The model under review builds one solid part; all positions refer to its coordinate system, in mm. A direction names the side the tool comes from. Give positions to 0.01 mm unless a question says otherwise; leave off trailing zeros. Write each loop counter-clockwise with the first axis right and the second up, starting at its lowest first coordinate (ties: lowest second). Pieces come first, ordered by that corner, then holes. Notation, with made-up numbers: (-9, -27) - (10, -27) arc R26 cw to (10, 1) - close; hole circle Ø9 at (-18, -37.75). An arc over 180 degrees is marked (long way). Write item = value, one per line.
```python
from build123d import *

# Parameters (mm, degrees)
F0_R     = 7.5
F2_DEPTH = 2
F3_DEPTH = 1


with BuildPart() as f2:
    # F0 (on Top) → F2 (new body)
    with BuildSketch(Plane.XY):
        Circle(F0_R)
    extrude(amount=-F2_DEPTH)

    # F1 (on Top) → F3 (join)
    with BuildSketch(Plane.XY):
        with BuildLine():
            add(Edge.make_bspline(
                [(0.0604885835, 7.3933677407), (0.3177365835, 6.9391977407), (0.5701195835, 6.4822377407), (0.8330605835, 6.0315707407)],
                knots=[0, 0, 0, 0, 1, 1, 1, 1], degree=3))
            add(Edge.make_bspline(
                [(-0.0762024165, 7.3933677407), (-0.0304464165, 7.3933677407), (0.0150095835, 7.3933677407), (0.0604885835, 7.3933677407)],
                knots=[0, 0, 0, 0, 1, 1, 1, 1], degree=3))
            add(Edge.make_bspline(
                [(-0.1212204165, 7.2902617407), (-0.1024804165, 7.3224177407), (-0.0909554165, 7.3588837407), (-0.0762024165, 7.3933677407)],
                knots=[0, 0, 0, 0, 1, 1, 1, 1], degree=3))
            add(Edge.make_bspline(
                [(-5.9762144165, -2.7421532593), (-4.0245564165, 0.6020177407), (-2.0726114165, 3.9459087407), (-0.1212204165, 7.2902617407)],
                knots=[0, 0, 0, 0, 1, 1, 1, 1], degree=3))
            add(Edge.make_bspline(
                [(-6.5031424165, -3.6556322593), (-6.3136034165, -3.3269782593), (-6.1463944165, -3.0337092593), (-5.9762144165, -2.7421532593)],
                knots=[0, 0, 0, 0, 1, 1, 1, 1], degree=3))
            add(Edge.make_bspline(
                [(6.4969945835, -3.6556322593), (2.1508305835, -3.6556322593), (-2.1525754165, -3.6556322593), (-6.5031424165, -3.6556322593)],
                knots=[0, 0, 0, 0, 1, 1, 1, 1], degree=3))
            add(Edge.make_bspline(
                [(6.3467955835, -3.3839732593), (6.3915375835, -3.4597902593), (6.4323375835, -3.5381272593), (6.4969945835, -3.6556322593)],
                knots=[0, 0, 0, 0, 1, 1, 1, 1], degree=3))
            add(Edge.make_bspline(
                [(5.4107935835, -1.7983302593), (5.7208275835, -2.3279572593), (6.0352405835, -2.8551552593), (6.3467955835, -3.3839732593)],
                knots=[0, 0, 0, 0, 1, 1, 1, 1], degree=3))
            add(Edge.make_bspline(
                [(0.8330605835, 6.0315707407), (2.3574805835, 3.4207877407), (3.8841375835, 0.8110887407), (5.4107935835, -1.7983302593)],
                knots=[0, 0, 0, 0, 1, 1, 1, 1], degree=3))
        make_face()
        with BuildLine():
            add(Edge.make_bspline(
                [(-5.7796534165, -3.2501722593), (-4.2207504165, -3.2501722593), (-2.7330644165, -3.2501722593), (-1.2455714165, -3.2501722593)],
                knots=[0, 0, 0, 0, 1, 1, 1, 1], degree=3))
            add(Edge.make_bspline(
                [(-3.3280754165, 0.9378677407), (-4.1345774165, -0.4399492593), (-4.9410894165, -1.8178682593), (-5.7796534165, -3.2501722593)],
                knots=[0, 0, 0, 0, 1, 1, 1, 1], degree=3))
            add(Edge.make_bspline(
                [(-1.2455714165, -3.2501722593), (-2.9605984165, -2.3525382593), (-3.6127754165, -0.9545362593), (-3.3280754165, 0.9378677407)],
                knots=[0, 0, 0, 0, 1, 1, 1, 1], degree=3))
        make_face(mode=Mode.SUBTRACT)
        with BuildLine():
            add(Edge.make_bspline(
                [(-0.2542014165, 3.0525277407), (-1.5089494165, 3.0320817407), (-2.9568184165, 1.8495517407), (-3.0198624165, 0.1261557407)],
                knots=[0, 0, 0, 0, 1, 1, 1, 1], degree=3))
            add(Edge.make_bspline(
                [(-0.2542014165, -3.0399232593), (-0.2542014165, -1.0090972593), (-0.2542014165, 1.0216117407), (-0.2542014165, 3.0525277407)],
                knots=[0, 0, 0, 0, 1, 1, 1, 1], degree=3))
            add(Edge.make_bspline(
                [(-3.0198624165, 0.1261557407), (-3.0896374165, -1.7814012593), (-1.4984154165, -3.0158812593), (-0.2542014165, -3.0399232593)],
                knots=[0, 0, 0, 0, 1, 1, 1, 1], degree=3))
        make_face(mode=Mode.SUBTRACT)
        with BuildLine():
            add(Edge.make_bspline(
                [(3.3546825835, 0.8849197407), (3.6216575835, -1.0009142593), (2.9443555835, -2.3765812593), (1.1968255835, -3.2457582593)],
                knots=[0, 0, 0, 0, 1, 1, 1, 1], degree=3))
            add(Edge.make_bspline(
                [(5.7743975835, -3.2457582593), (4.9505145835, -1.8388482593), (4.1524725835, -0.4769692593), (3.3546825835, 0.8849197407)],
                knots=[0, 0, 0, 0, 1, 1, 1, 1], degree=3))
            add(Edge.make_bspline(
                [(1.1968255835, -3.2457582593), (2.7469015835, -3.2457582593), (4.2381755835, -3.2457582593), (5.7743975835, -3.2457582593)],
                knots=[0, 0, 0, 0, 1, 1, 1, 1], degree=3))
        make_face(mode=Mode.SUBTRACT)
        with BuildLine():
            add(Edge.make_bspline(
                [(0.2117715835, 3.0732277407), (0.2032195835, 2.9602327407), (0.1901495835, 2.8641567407), (0.1898735835, 2.7679887407)],
                knots=[0, 0, 0, 0, 1, 1, 1, 1], degree=3))
            add(Edge.make_bspline(
                [(1.7295995835, 2.5419747407), (1.2838885835, 2.8565037407), (0.7887565835, 3.0489087407), (0.2117715835, 3.0732277407)],
                knots=[0, 0, 0, 0, 1, 1, 1, 1], degree=3))
            add(Edge.make_bspline(
                [(2.9614815835, -0.7022442593), (3.2517605835, 0.5176517407), (2.7668865835, 1.8099267407), (1.7295995835, 2.5419747407)],
                knots=[0, 0, 0, 0, 1, 1, 1, 1], degree=3))
            add(Edge.make_bspline(
                [(0.4320915835, -3.0458662593), (1.6893525835, -2.8326462593), (2.6694735835, -1.9292522593), (2.9614815835, -0.7022442593)],
                knots=[0, 0, 0, 0, 1, 1, 1, 1], degree=3))
            add(Edge.make_bspline(
                [(0.1763655835, -2.8243612593), (0.1757435835, -3.0158812593), (0.2339925835, -3.0793612593), (0.4320915835, -3.0458662593)],
                knots=[0, 0, 0, 0, 1, 1, 1, 1], degree=3))
            add(Edge.make_bspline(
                [(0.1898735835, 2.7679887407), (0.1853785835, 0.9039367407), (0.1838565835, -0.9602062593), (0.1763655835, -2.8243612593)],
                knots=[0, 0, 0, 0, 1, 1, 1, 1], degree=3))
        make_face(mode=Mode.SUBTRACT)
        with BuildLine():
            add(Edge.make_bspline(
                [(-2.3909204165, 2.5383797407), (-2.3739784165, 2.5269457407), (-2.3571514165, 2.5151437407), (-2.3404854165, 2.5037107407)],
                knots=[0, 0, 0, 0, 1, 1, 1, 1], degree=3))
            add(Edge.make_bspline(
                [(-0.3082324165, 6.1343087407), (-1.0024544165, 4.9357577407), (-1.6968604165, 3.7371147407), (-2.3909204165, 2.5383797407)],
                knots=[0, 0, 0, 0, 1, 1, 1, 1], degree=3))
            add(Edge.make_bspline(
                [(-0.2558374165, 6.1257567407), (-0.2732874165, 6.1285457407), (-0.2908514165, 6.1315197407), (-0.3082324165, 6.1343087407)],
                knots=[0, 0, 0, 0, 1, 1, 1, 1], degree=3))
            add(Edge.make_bspline(
                [(-0.2339394165, 5.9442317407), (-0.2341234165, 6.0047397407), (-0.2481844165, 6.0652487407), (-0.2558374165, 6.1257567407)],
                knots=[0, 0, 0, 0, 1, 1, 1, 1], degree=3))
            add(Edge.make_bspline(
                [(-0.2276464165, 3.6721807407), (-0.2339394165, 4.4295387407), (-0.2315194165, 5.1869657407), (-0.2339394165, 5.9442317407)],
                knots=[0, 0, 0, 0, 1, 1, 1, 1], degree=3))
            add(Edge.make_bspline(
                [(-0.4507784165, 3.4107147407), (-0.2747394165, 3.4329587407), (-0.2261024165, 3.5076897407), (-0.2276464165, 3.6721807407)],
                knots=[0, 0, 0, 0, 1, 1, 1, 1], degree=3))
            add(Edge.make_bspline(
                [(-2.2525234165, 2.5683687407), (-1.7367614165, 3.0309067407), (-1.1393294165, 3.3233747407), (-0.4507784165, 3.4107147407)],
                knots=[0, 0, 0, 0, 1, 1, 1, 1], degree=3))
            add(Edge.make_bspline(
                [(-2.3404854165, 2.5037107407), (-2.3110494165, 2.5251477407), (-2.2792624165, 2.5439577407), (-2.2525234165, 2.5683687407)],
                knots=[0, 0, 0, 0, 1, 1, 1, 1], degree=3))
        make_face(mode=Mode.SUBTRACT)
        with BuildLine():
            add(Edge.make_bspline(
                [(2.3211755835, 2.5607157407), (2.3334385835, 2.5692677407), (2.3453105835, 2.5780037407), (2.3572965835, 2.5865557407)],
                knots=[0, 0, 0, 0, 1, 1, 1, 1], degree=3))
            add(Edge.make_bspline(
                [(1.6364045835, 3.0178597407), (1.8710625835, 2.8758667407), (2.0933875835, 2.7136807407), (2.3211755835, 2.5607157407)],
                knots=[0, 0, 0, 0, 1, 1, 1, 1], degree=3))
            add(Edge.make_bspline(
                [(0.3738415835, 3.4342957407), (0.8199905835, 3.3685777407), (1.2488745835, 3.2528627407), (1.6364045835, 3.0178597407)],
                knots=[0, 0, 0, 0, 1, 1, 1, 1], degree=3))
            add(Edge.make_bspline(
                [(0.2013985835, 3.5821437407), (0.2018595835, 3.5301877407), (0.3079165835, 3.4442077407), (0.3738415835, 3.4342957407)],
                knots=[0, 0, 0, 0, 1, 1, 1, 1], degree=3))
            add(Edge.make_bspline(
                [(0.1935845835, 6.1167437407), (0.1935845835, 5.2718847407), (0.1904265835, 4.4270257407), (0.2013985835, 3.5821437407)],
                knots=[0, 0, 0, 0, 1, 1, 1, 1], degree=3))
            add(Edge.make_bspline(
                [(0.2710125835, 6.1454647407), (0.2450795835, 6.1359217407), (0.2194245835, 6.1263787407), (0.1935845835, 6.1167437407)],
                knots=[0, 0, 0, 0, 1, 1, 1, 1], degree=3))
            add(Edge.make_bspline(
                [(2.3572965835, 2.5865557407), (1.6618995835, 3.7728667407), (0.9663175835, 4.9591547407), (0.2710125835, 6.1454647407)],
                knots=[0, 0, 0, 0, 1, 1, 1, 1], degree=3))
        make_face(mode=Mode.SUBTRACT)
    extrude(amount=F3_DEPTH)


solid = f2.part
```
1. For line 1 (Y direction, x = 0.5, z = 0.75); line 2 (Y direction, x = 2.75, z = 0.8); line 3 (Z direction, x = -1.75, y = 5.5), list the stretches that pass through material, from the lowest coordinate up. Write a range as from..to.
Findings below:
line_1 = -3.66..-3.03, 3.05..3.41, 5.75..6.61
line_2 = -3.66..-3.25, -2.01..-1.31, 1.32..2.75
line_3 = -2..0
2. Take a section at A-A on y = -4.5. Give the boundary of the cut face in (x, z), and give its area (3 significant figures).
Findings below:
outline = (-6, -2) - (6, -2) - (6, 0) - (-6, 0) - close
area = 24.0 mm²
3. Machinability: for faces 1 (the flat face through (0, 0, -2)), 2 (the flat face through (1, 4, 0)), which of the approach directions +Z, -Z, +X, -X, +Y, -Y give a long, thin tool a straight path to every point of the face, cutting with its end or side? Answer none if there is none.
Findings below:
face_1 = -Z, +X, -X, +Y, -Y
face_2 = +Z
4. Draft analysis for pull direction X (two halves, no side actions). For faces 3 (the flat face through (0, 0, 1)), 4 (the cylindrical face through (-7.493, 0.33, -0.986)), 5 (the flat face through (4, -2, 0)), state which applies: +X half, -X half, draft (parallel to the pull), parting line (faces both ways), or undercut.
Findings below:
face_3 = draft
face_4 = parting line
face_5 = undercut
5. Insertion check: P1, Ø1, axis at y = -5.5, z = 0, coming from the +X side; P2, Ø2.5, axis at x = 1.5, y = 0, coming from the +Z side; P3, Ø1.5, axis at x = -2.5, z = 0.5, coming from the +Y side. Each pin has a flat end and moves straight along its axis. Give the tip position at first contact, or say it passes through.
Findings below:
P1 = 5.59
P2 = 0
P3 = 7.24
